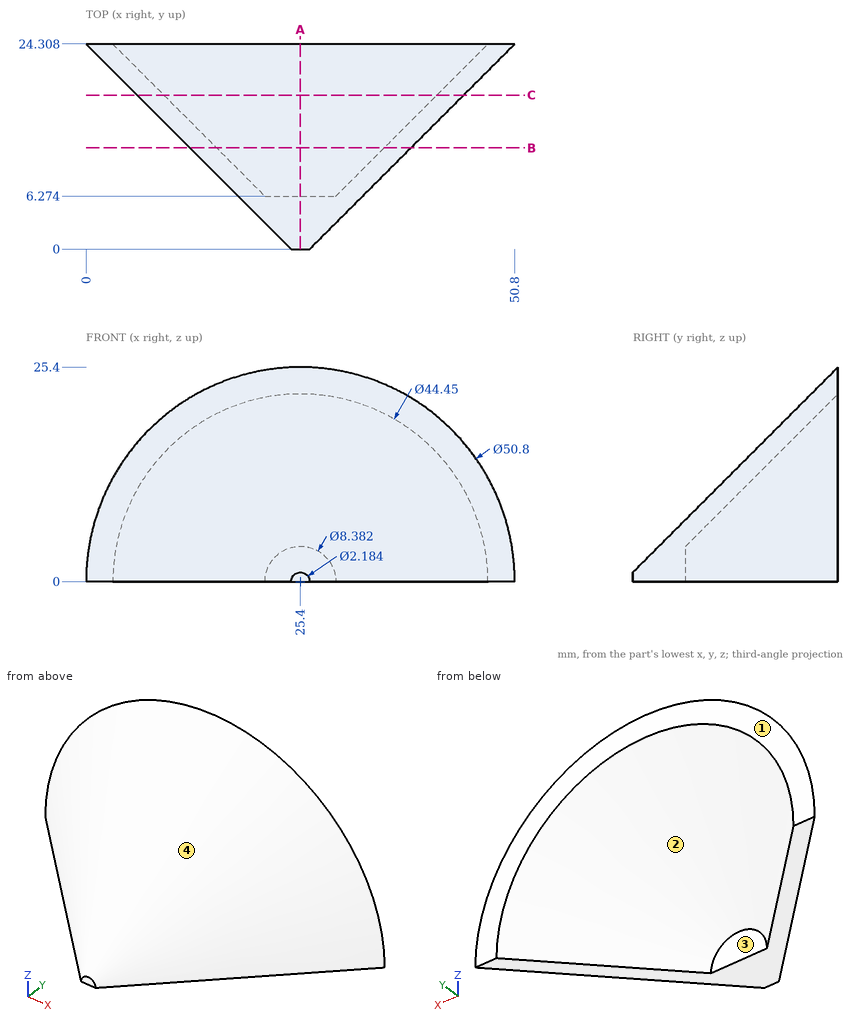
Check sheet for the drawn part. Datum: minimum x, y, z corner. Units: mm. Round coordinates to 2 decimals unless told otherwise and drop trailing zeros. Order: outer loops, then holes, each group sorted by start corner. A loop starts at its lowest first (then second) coordinate and runs counter-clockwise, first axis right, second up.
1. Section check B-B on y = 12. Record the cut outline in (x, z) (1 decimal), then the cut area to 3 significant figures.
Final values:
outline: (12.3, 0) - (15.5, 0) arc R9.9 cw to (35.3, 0) - (38.5, 0) arc R13.1 ccw to start
area: 115 mm2
2. Thickness scan on L1, parallel to X at y = 23, z = 2.25 (1 decimal); L2, parallel to X at y = 12.5, z = 6.25 (1 decimal); L3, parallel to Z at x = 21, y = 8.25. Record the ranges inside material, lowest first.
Final values:
L1: x = 1.4 to 4.6, 46.2 to 49.4
L2: x = 13.3 to 17.1, 33.7 to 37.5
L3: z = 4.32 to 8.24
3. Release check for a two-part mould opening along X. For the marked faces 1, 2, 3 and 4 record: +X half, -X half, draft (parallel to the pull), parting line (faces both ways), or undercut.
Final values:
face 1: draft
face 2: undercut
face 3: undercut
face 4: parting line
4. Go/stop test with flat-tipped pins: P1, Ø2, axis at x = 17, z = 18.5, coming from the +Y side; P2, Ø1.5, axis at y = 20.5, z = 16, coming from the -X side (1 decimal); P3, Ø1, axis at x = 25.5, z = 21.5, coming from the -Y side. Record where each tip stops, or that it passes through.
Final values:
P1: stops at y = 23.4
P2: stops at x = 9.6
P3: stops at y = 19.91
5. Section check A-A on x = 25.4. Record the cut outline in (y, z) (1 decimal).
Final values:
outline: (0, 0) - (6.3, 0) - (6.3, 4.2) - (24.3, 22.2) - (24.3, 25.4) - (0, 1.1) - close
6. Section check C-C on y = 18.25. Record the cut outline in (x, z) (1 decimal).
Final values:
outline: (6.1, 0) - (9.2, 0) arc R16.2 cw to (41.6, 0) - (44.7, 0) arc R19.3 ccw to start
